Work out the finished part from the listing and answer in its coordinate system (mm). A direction names the side the tool comes from. Round coordinates to 2 decimals unless told otherwise and drop trailing zeros. Write each loop counter-clockwise with the first axis right and the second up, starting at its lowest first coordinate (ties: lowest second). Pieces come first, ordered by that corner, then holes. Notation, with made-up numbers: M 4,17 L 47,17 A26 cw 47,45 Z; hole C -29.5,68.25 d3. An arc over 180 degrees is marked long. Answer in a Markdown table with one row per item.
```python
from build123d import *

# Parameters (mm, degrees)
F0_W     = 76.2
F0_H     = 76.2
F1_DEPTH = 76.2
F3_T     = -2.54
F2_W     = 76.2
F2_H     = 76.2
F2_W_2   = 17.78
F2_H_2   = 17.78
F4_DEPTH = 76.2
F5_DEPTH = 63.5


with BuildPart() as f1:
    # F0 (on Top) → F1 (new body)
    with BuildSketch(Plane.XY):
        Rectangle(F0_W, F0_H)
    extrude(amount=F1_DEPTH)

    # F3
    f3_openings = [f1.faces().sort_by_distance(p)[0] for p in [
        (38.1, 0, 38.1),
    ]]
    offset(amount=F3_T, openings=f3_openings)

    # F2 (on face) → F4 (join)
    with BuildSketch(Plane.YZ.offset(38.1)):
        with Locations((0, 38.1)):
            Rectangle(F2_W, F2_H)
        Polygon((-8.5432641208, 30.0269989133), (-8.5432641208, 36.3769989133), (1.6167358792, 36.3769989133), (1.6167358792, 30.0269989133), (13.0484727508, 30.0269989133), (13.0484727508, 23.6769989133), (13.0484727508, 17.3269989133), (13.0484727508, 10.5390315875), (6.3009303994, 10.5390315875), (6.3009303994, 17.3269989133), (-12.8088379279, 17.3269989133), (-12.8088379279, 10.5390315875), (-19.9750009924, 10.5390315875), (-19.9750009924, 17.3269989133), (-19.9750009924, 23.6769989133), (-19.9750009924, 30.0269989133), align=None, mode=Mode.SUBTRACT)
        with Locations((-15.9198542664, 59.1702901899)):
            Rectangle(F2_W_2, F2_H_2, mode=Mode.SUBTRACT)
        with Locations((12.2508332058, 59.1702901899)):
            Rectangle(F2_W_2, F2_H_2, mode=Mode.SUBTRACT)
    extrude(amount=-F4_DEPTH)

    # F5 (add): faces of the model
    f5_faces = [f1.faces().sort_by_distance(p)[0] for p in [
        (-35.56, -15.9198542664, 59.1702901899),
        (-35.56, 12.2508332058, 59.1702901899),
    ]]
    extrude(f5_faces, amount=F5_DEPTH)


solid = f1.part
```
1. Consider line 1 along Y through (x, z) = (28, 59.5); line 2 along Z through (x, y) = (30, -17.5); line 3 along Z through (x, y) = (12.5, -17.5). Determine where each line is inside the solid, lowest interval first. Write a range as from..to.
Calculated:
| item | result |
|---|---|
| line 1 | y = -38.1..-24.81, -7.03..3.36, 21.14..38.1 |
| line 2 | z = 0..10.54, 30.03..50.28, 68.06..76.2 |
| line 3 | z = 0..10.54, 30.03..76.2 |
2. The part is cut by section D-D (y = -4). Determine the outline of the cut face in (x, z).
Calculated:
| item | result |
|---|---|
| outline | M -38.1,0 L 38.1,0 L 38.1,17.33 L -35.56,17.33 L -35.56,36.38 L 38.1,36.38 L 38.1,76.2 L -38.1,76.2 Z |
3. Given pin 1 (9 mm diameter, centred on y = -15.5, z = 61, fed in from +X); pin 2 (19.5 mm diameter, centred on y = 10.5, z = 63, fed in from +X), each flat-ended and moving along its own axis, determine where each tip first touches the part or whether it passes through.
Calculated:
| item | result |
|---|---|
| pin 1 | stops at x = 27.94 |
| pin 2 | stops at x = 38.1 |
4. Determine the mould class of faces 3 (the flat face through (-1, 38.1, 38)), 4 (the flat face through (33, -7.03, 59)), 5 (the flat face through (-1, 1, 76.2)) for opening direction Y: released by +Y, released by -Y, zero draft, split by the parting line, or undercut.
Calculated:
| item | result |
|---|---|
| face 3 | released by +Y |
| face 4 | undercut |
| face 5 | zero draft |
5. The part is cut by section B-B (y = 5). Determine the outline of the cut face in (x, z), plus the area to 3 significant figures.
Calculated:
| item | result |
|---|---|
| outline | M -38.1,0 L 38.1,0 L 38.1,17.33 L -35.56,17.33 L -35.56,30.03 L 38.1,30.03 L 38.1,50.28 L 27.94,50.28 L 27.94,68.06 L 38.1,68.06 L 38.1,76.2 L -38.1,76.2 Z |
| area | 4,690 mm² |
6. The part is cut by section C-C (y = 14.5). Determine the outline of the cut face in (x, z).
Calculated:
| item | result |
|---|---|
| outline | M -38.1,0 L 38.1,0 L 38.1,50.28 L 27.94,50.28 L 27.94,68.06 L 38.1,68.06 L 38.1,76.2 L -38.1,76.2 Z |
7. The part is cut by section A-A (x = 4). Determine the outline of the cut face in (y, z) (3 decimals), plus the area to 3 significant figures.
Calculated:
| item | result |
|---|---|
| outline | M -38.1,0 L 38.1,0 L 38.1,76.2 L -38.1,76.2 Z; hole M -19.975,10.539 L -12.809,10.539 L -12.809,17.327 L 6.301,17.327 L 6.301,10.539 L 13.048,10.539 L 13.048,30.027 L 1.617,30.027 L 1.617,36.377 L -8.543,36.377 L -8.543,30.027 L -19.975,30.027 Z |
| area | 5,230 mm² |
8. A tool of negligible diameter and unlimited length cuts with its end or side. For faces 1 (the flat face through (2, -14, 30.027)), 2 (the flat face through (-38.1, -1, 38)), from which of +Z, -Z, +X, -X, +Y, -Y can it reach the whole face along a straight path? Write none if from no direction.
Calculated:
| item | result |
|---|---|
| face 1 | +X |
| face 2 | +Z, -Z, -X, +Y, -Y |
